Autodesk Inventor part; units mm, degrees
ref_plane "YZ Plane" through (0, 0, 0) normal (1, 0, 0) x (0, 1, 0)
ref_plane "XZ Plane" through (0, 0, 0) normal (0, 1, 0) x (-1, 0, 0)
ref_plane "XY Plane" through (0, 0, 0) normal (0, 0, 1) x (1, 0, 0)
sketch "Skizze1" plane through (0, 0, 0) normal (0, 1, 0) x (-1, 0, 0)
  circle A0 centre (0, 0) radius 13
  dimension "d0" = 26
extrude "Extrusion1" add sketch "Skizze1" along normal blind 6
sketch "Skizze2" plane through (0, 0, 0) normal (0, -1, 0) x (1, 0, 0)
  circle A0 centre (0, 0) radius 3
  dimension "d3" = 6
extrude "Extrusion2" add sketch "Skizze2" along normal blind 32
sketch "Skizze3" plane through (0, 0, 0) normal (0, 1, 0) x (1, 0, 0)
  circle A0 centre (-9.5, 0) radius 1.5
  point P0 (0, 0)
  dimension "d6" = 3
  dimension "d7" = 9.5
extrude "Extrusion3" add sketch "Skizze3" along normal blind 13.5
fillet "Rundung1" radius 1 2 edges at (13, 0, 0) (13, 6, 0)
properties part number "handle" material "Stahl, weich"
The model under review builds one solid part; all positions refer to its coordinate system, in mm. A direction names the side the tool comes from. Round coordinates to 2 decimals unless told otherwise and drop trailing zeros. Loops run counter-clockwise (first coordinate to the right, second up) from the corner with the lowest first, then second, coordinate; pieces in that order, holes last.
Item 1: Take a section at A-A (x = 0). Write out the cut boundary in (y, z).
Determined:
outline: (-32, -3) - (0, -3) - (0, -12) arc R1 ccw to (1, -13) - (5, -13) arc R1 ccw to (6, -12) - (6, 12) arc R1 ccw to (5, 13) - (1, 13) arc R1 ccw to (0, 12) - (0, 3) - (-32, 3) - close
Item 2: Clearance check with flat-ended pins moving along their axes: pin 1 Ø8 at (y, z) = (3.5, -8.5) entering from -X; pin 2 Ø12 at (x, z) = (-1.5, -1.5) entering from +Y; pin 3 Ø3 at (x, z) = (-9.5, -2.5) entering from -Y. State where each tip first meets the part, or that it passes through.
Determined:
pin 1: stops at x = -12.2
pin 2: stops at y = 6
pin 3: stops at y = 0
Item 3: For line 1 (Y direction, x = 1.5, z = -8.75); line 2 (X direction, y = 2, z = 0.5); line 3 (Z direction, x = 0.25, y = -12), list the stretches that pass through material, from the lowest coordinate up.
Determined:
line 1: y = 0 to 6
line 2: x = -12.99 to 12.99
line 3: z = -2.99 to 2.99
Item 4: Take a section at C-C (y = -4). Write out the cut boundary in (x, z), then the cut area to 3 significant figures.
Determined:
outline: circle Ø6 at (0, 0)
area: 28.3 mm2
Item 5: For faces 1 (the face through (-3, -16, 0)), 2 (the face through (-10, 13.5, 0)), 3 (the face through (-11, 10, 0)), list the 3-axis set-ups (+Z, -Z, +X, -X, +Y, -Y) from which the entire face can be reached by the end or side of a thin tool; tool diameter is ignored.
Determined:
face 1: -Y
face 2: +Z, -Z, +X, -X, +Y
face 3: +Y
Item 6: Take a section at B-B (z = 0). Write out the cut boundary in (x, y), then the cut area to 3 significant figures.
Determined:
outline: (-13, 1) arc R1 ccw to (-12, 0) - (-3, 0) - (-3, -32) - (3, -32) - (3, 0) - (12, 0) arc R1 ccw to (13, 1) - (13, 5) arc R1 ccw to (12, 6) - (-8, 6) - (-8, 13.5) - (-11, 13.5) - (-11, 6) - (-12, 6) arc R1 ccw to (-13, 5) - close
area: 370 mm2
